Source: CAD feature listing. Evaluate the final solid. Frame: model axes, mm. Face numbers are marked on the shaded views. A direction names the side the tool comes from. Round coordinates to 2 decimals unless told otherwise and drop trailing zeros. Loops run counter-clockwise (first coordinate to the right, second up) from the corner with the lowest first, then second, coordinate; pieces in that order, holes last. Notation, with made-up numbers: M -23.5,38 L 14.5,38 A4 ccw 14.5,43 Z; hole C 64.25,-4.75 d9. An arc over 180 degrees is marked long. Answer as CSV lines item,"result". Start each with the question number.
```python
from build123d import *

# Parameters (mm, degrees)
BOSS_EXTRUDE1_DEPTH = 12
SKETCH2_R           = 2.5
CUT_EXTRUDE1_DEPTH  = 13
SKETCH3_W           = 217
SKETCH3_H           = 87
BOSS_EXTRUDE2_DEPTH = 285


with BuildPart() as part:
    # Sketch1 → Boss-Extrude1 (new body)
    with BuildSketch(Plane.XY):
        Polygon((-108.5, 149), (108.5, 149), (108.5, -107), (108.5, -149), (-108.5, -149), (-108.5, -107), align=None)
    extrude(amount=BOSS_EXTRUDE1_DEPTH)

    # Sketch2 → Cut-Extrude1 (cut, through all)
    with BuildSketch(Plane(origin=(0, 0, 0), x_dir=(-1, 0, 0), z_dir=(0, 0, -1))):
        with Locations((0, 134)):
            Circle(SKETCH2_R)
    extrude(amount=-CUT_EXTRUDE1_DEPTH, mode=Mode.SUBTRACT)

    # Sketch3 → Boss-Extrude2 (add)
    with BuildSketch(Plane(origin=(0, 0, 0), x_dir=(-1, 0, 0), z_dir=(0, 0, -1))):
        with Locations((0, -105.5)):
            Rectangle(SKETCH3_W, SKETCH3_H)
    extrude(amount=BOSS_EXTRUDE2_DEPTH)


solid = part.part
```
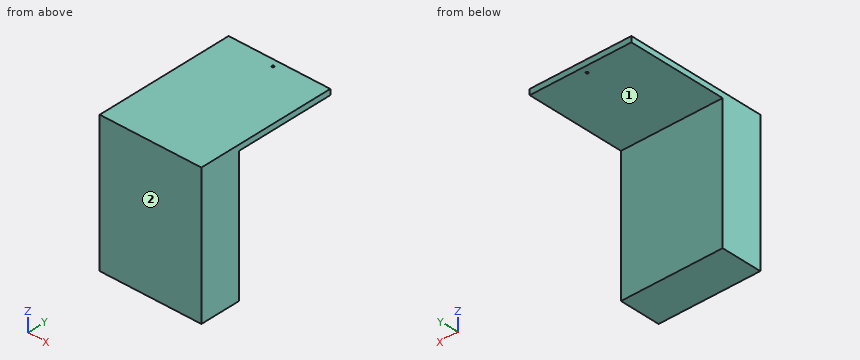
1) Section B-B, the plane y = -3.5. Return loops of the section in (x, z).
2) Access query for the marked faces 1 and 2. Directions: +Z, -Z, +X, -X, +Y, -Y. A direction counts if a zero-diameter tool reaches every point of the face in a straight line with its end or side. Return the directions, or none.
3) Section A-A, the plane x = -92. Return loops of the section in (y, z), and give its area (3 significant figures).
4) Contact query for flat-ended pins moving along their axis: pin 1 Ø1 at (x, z) = (76.5, -233.5) entering from +Y; pin 2 Ø3 at (x, y) = (0, 134) entering from +Z; pin 3 Ø4 at (x, y) = (-45, 103.5) entering from -Z. Output: stop coordinate, or through.
5) Ray query, line 1 along X through (y, z) = (134, 9); line 2 along Y through (x, z) = (0, 4); line 3 along Z through (x, y) = (57.5, 82). Return the intervals inside material, ascending.
6) Section C-C, the plane z = -173. Return loops of the section in (x, y).
Findings below:
1,outline,"M -108.5,0 L 108.5,0 L 108.5,12 L -108.5,12 Z"
2,face 1,"-Z, +X, -X, +Y"
2,face 2,"+Z, -Z, +X, -X, -Y"
3,outline,"M -149,-285 L -62,-285 L -62,0 L 149,0 L 149,12 L -149,12 Z"
3,area,"28,400 mm²"
4,pin 1,"y = -62"
4,pin 2,"through"
4,pin 3,"z = 0"
5,line 1,"-108.5 to -2.5, 2.5 to 108.5"
5,line 2,"-149 to 131.5, 136.5 to 149"
5,line 3,"0 to 12"
6,outline,"M -108.5,-149 L 108.5,-149 L 108.5,-62 L -108.5,-62 Z"
